Geometry check sheet. Reference: the model listing, model coordinates, mm. A direction names the side the tool comes from. Round coordinates to 2 decimals unless told otherwise and drop trailing zeros. Order: outer loops, then holes, each group sorted by start corner. A loop starts at its lowest first (then second) coordinate and runs counter-clockwise, first axis right, second up.
(1) Cross-section at B-B on y = 1. Enter the section's corners in (x, z), and give its area (3 significant figures).
(2) Draft check along Z on faces 1 (the face through (4.563, 7.905, -0.867)), 2 (the face through (-2, -7, 0)), 3 (the face through (0, 0, 2)). Enter one of: pulls with the +Z half, pulls with the -Z half, needs draft (parallel to the pull), parting line crosses it, or undercut.
(3) Gauge pin test, flat ends, axial feed: P1, Ø1.5, axis at x = 6.5, y = 10, coming from the +Z side; P2, Ø1.5, axis at x = 5.5, y = 1, coming from the -Z side; P3, Ø2, axis at y = 1, z = -9.5, coming from the -X side. Record the tip position at first contact, or that the pin passes through.
(4) Thickness scan on L1, parallel to Y at x = 4.5, z = 0; L2, parallel to X at y = 0, z = 3.5; L3, parallel to Z at x = 7.25, y = 4. Record the ranges inside material, lowest first.
(5) Cross-section at D-D on y = -8. Enter the section's corners in (x, z).
(6) Set-up check for faces 4 (the face through (3.04, 4.38, -8.43)), 5 (the face through (-5, -6, 0)): record each of +Z, -Z, +X, -X, +Y, -Y from which the full face is reachable in a straight line by a thin tool's end or side.
(7) Cross-section at A-A on z = 0. Enter the section's corners in (x, y), and give its area (3 significant figures).
(8) Cross-section at C-C on x = 4. Enter the section's corners in (y, z), and give its area (3 significant figures).
Autodesk Inventor part; units mm, degrees
ref_plane "YZ Plane" through (0, 0, 0) normal (1, 0, 0) x (0, 1, 0)
ref_plane "XZ Plane" through (0, 0, 0) normal (0, 1, 0) x (-1, 0, 0)
ref_plane "XY Plane" through (0, 0, 0) normal (0, 0, 1) x (1, 0, 0)
sketch "Sketch1" plane through (0, 0, 0) normal (0, 0, 1) x (1, 0, 0)
  line L0 (0, 0) -> (0, 9.5)
  line L1 (0, 9.5) -> (6, 9.5)
  line L2 (6, 9.5) -> (6, 12.5)
  line L3 (6, 12.5) -> (9, 12.5)
  line L4 (9, 12.5) -> (9, 0)
  line L5 (9, 0) -> (0, 0)
  point P0 (7.5, 12.5)
  dimension "d0" = 3
  dimension "d1" = 6
  dimension "d2" = 25
  dimension "d3" = 19
revolve "Revolution1" add sketch "Sketch1" angle 360 about axis through (9, 0, 0) along (-1, 0, 0)
sketch "Sketch2" plane through (0, 0, 0) normal (-1, 0, 0) x (0, 0, 1)
  point P0 (0, 0)
  point P1 (0, 4)
  dimension "d12" = 4
hole "Hole1" at (0, 4, 0) direction (1, 0, 0) diameter 8 depth 9
sketch "Sketch4" plane through (0, 0, 0) normal (-1, 0, 0) x (0, 0, 1)
  circle A0 centre (0, -6) radius 1
  point P0 (0, 0)
  dimension "d21" = 6
  dimension "d22" = 2
extrude "Extrusion1" add sketch "Sketch4" along normal blind 5
properties part number "203"
Found:
1. outline: (0, -9.45) - (6, -9.45) - (6, -12.46) - (9, -12.46) - (9, -2.65) - (0, -2.65) - close; (0, 2.65) - (9, 2.65) - (9, 12.46) - (6, 12.46) - (6, 9.45) - (0, 9.45) - close
1. area: 141 mm2
2. face 1: undercut
2. face 2: parting line crosses it
2. face 3: needs draft
3. P1: stops at z = 8.41
3. P2: stops at z = -12.49
3. P3: stops at x = 0
4. L1: y = -9.5 to 0, 8 to 9.5
4. L2: x = 0 to 9
4. L3: z = -11.84 to -4, 4 to 11.84
5. outline: (0, -5.12) - (6, -5.12) - (6, -9.6) - (9, -9.6) - (9, 9.6) - (6, 9.6) - (6, 5.12) - (0, 5.12) - close
6. face 4: -X
6. face 5: +Z, -Z, -X, +Y, -Y
7. outline: (-5, -7) - (0, -7) - (0, -9.5) - (6, -9.5) - (6, -12.5) - (9, -12.5) - (9, 0) - (0, 0) - (0, -5) - (-5, -5) - close; (0, 8) - (9, 8) - (9, 12.5) - (6, 12.5) - (6, 9.5) - (0, 9.5) - close
7. area: 127 mm2
8. outline: circle Ø19 at (0, 0); hole circle Ø8 at (4, 0)
8. area: 233 mm2
